from build123d import *

# Parameters (mm, degrees)
F0_W     = 15
F0_H     = 15
F0_R     = 4.955
F1_DEPTH = 7.5
F2_R     = 2.5
F3_DEPTH = 1.5
F4_R     = 2.5
F5_DEPTH = 1.5
F6_R     = 2.5
F7_DEPTH = 1.5
F8_R     = 2.5
F9_DEPTH = 1.5


with BuildPart() as f1:
    # F0 (on Top) → F1 (new body, symmetric)
    with BuildSketch(Plane.XY):
        Rectangle(F0_W, F0_H)
        Circle(F0_R, mode=Mode.SUBTRACT)
    extrude(amount=F1_DEPTH, both=True)

    # F2 (on face) → F3 (join)
    with BuildSketch(Plane(origin=(0, 7.5, 0), x_dir=(-1, 0, 0), z_dir=(0, 1, 0))):
        Circle(F2_R)
    extrude(amount=F3_DEPTH)

    # F4 (on face) → F5 (cut)
    with BuildSketch(Plane.XZ.offset(7.5)):
        Circle(F4_R)
    extrude(amount=-F5_DEPTH, mode=Mode.SUBTRACT)

    # F6 (on face) → F7 (cut)
    with BuildSketch(Plane.YZ.offset(7.5)):
        Circle(F6_R)
    extrude(amount=-F7_DEPTH, mode=Mode.SUBTRACT)

    # F8 (on face) → F9 (cut)
    with BuildSketch(Plane(origin=(-7.5, 0, 0), x_dir=(0, -1, 0), z_dir=(-1, 0, 0))):
        Circle(F8_R)
    extrude(amount=-F9_DEPTH, mode=Mode.SUBTRACT)


solid = f1.part
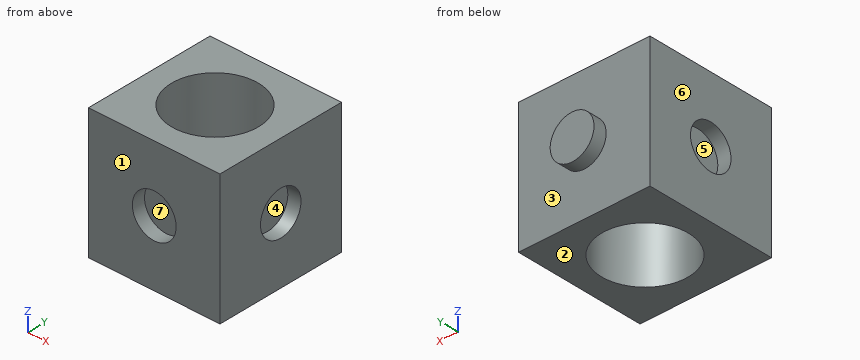
Read the model definition and answer for the solid it produces. Units are mm, in the model's axes. Face numbers are marked on the shaded views. A direction names the side the tool comes from. Coordinates: 2 decimals unless noted, no trailing zeros. Order: outer loops, then holes, each group sorted by start corner. A loop starts at its lowest first (then second) coordinate and runs counter-clockwise, first axis right, second up. Notation, with made-up numbers: M 35,-24.75 L 71,-24.75 A5 cw 71,-20.75 Z; hole C 83.25,88.25 d3. An arc over 180 degrees is marked long. Put each result on its own line as item: value. Start each with the question number.
Item 1: For the marked faces 5, 6 and 7, determine the directions among +Z, -Z, +X, -X, +Y, -Y from which every point of the face is accessible in a straight line to the end or side of a thin tool.
Item 2: Given pin 1 Ø4 at (y, z) = (0, 0) entering from +X; pin 2 Ø9 at (x, y) = (0, 0) entering from +Z; pin 3 Ø1 at (x, z) = (-3.5, -4.5) entering from +Y; pin 4 Ø1.5 at (y, z) = (1, 0.5) entering from -X, each flat-ended and moving along its own axis, determine where each tip first touches the part or whether it passes through.
Item 3: Section B-B, the plane y = 0 is taken. Determine the outline of the cut face in (x, z) (3 decimals).
Item 4: Section D-D, the plane y = -3 is taken. Determine the outline of the cut face in (x, z), plus the area to 3 significant figures.
Item 5: Section C-C, the plane x = 0 is taken. Determine the outline of the cut face in (y, z) (3 decimals), plus the area to 4 significant figures.
Item 6: Section A-A, the plane z = 0 is taken. Determine the outline of the cut face in (x, y) (3 decimals), plus the area to 3 significant figures.
Item 7: The mould has two halves that part along Y. Classify the marked faces 1, 2, 3 and 4: +Y half, -Y half, draft (parallel to the pull), parting line (faces both ways), or undercut.
Item 8: Consider probe 1 along Z at (x, y) = (-6.8, 0); probe 2 along Y at (x, z) = (0, -2) (3 decimals); probe 3 along X at (y, z) = (1.75, -0.25). Determine where each line is inside the solid, lowest interval first. Write a range as [from, to].
Computed:
1. face 5: -X
1. face 6: +Z, -Z, -X, +Y, -Y
1. face 7: -Y
2. pin 1: stops at x = 6
2. pin 2: passes through
2. pin 3: stops at y = 7.5
2. pin 4: stops at x = -6
3. outline: M -7.5,-7.5 L -4.955,-7.5 L -4.955,7.5 L -7.5,7.5 L -7.5,2.5 L -6,2.5 L -6,-2.5 L -7.5,-2.5 Z; M 4.955,-7.5 L 7.5,-7.5 L 7.5,-2.5 L 6,-2.5 L 6,2.5 L 7.5,2.5 L 7.5,7.5 L 4.955,7.5 Z
4. outline: M -7.5,-7.5 L -3.94,-7.5 L -3.94,7.5 L -7.5,7.5 Z; M 3.94,-7.5 L 7.5,-7.5 L 7.5,7.5 L 3.94,7.5 Z
4. area: 107 mm2
5. outline: M -7.5,-7.5 L -4.955,-7.5 L -4.955,7.5 L -7.5,7.5 L -7.5,2.5 L -6,2.5 L -6,-2.5 L -7.5,-2.5 Z; M 4.955,-7.5 L 7.5,-7.5 L 7.5,-2.5 L 9,-2.5 L 9,2.5 L 7.5,2.5 L 7.5,7.5 L 4.955,7.5 Z
5. area: 76.35 mm2
6. outline: M -7.5,-7.5 L -2.5,-7.5 L -2.5,-6 L 2.5,-6 L 2.5,-7.5 L 7.5,-7.5 L 7.5,-2.5 L 6,-2.5 L 6,2.5 L 7.5,2.5 L 7.5,7.5 L 2.5,7.5 L 2.5,9 L -2.5,9 L -2.5,7.5 L -7.5,7.5 L -7.5,2.5 L -6,2.5 L -6,-2.5 L -7.5,-2.5 Z; hole C 0,0 d9.91
6. area: 133 mm2
7. face 1: -Y half
7. face 2: draft
7. face 3: +Y half
7. face 4: undercut
8. probe 1: z = [-7.5, -2.5], [2.5, 7.5]
8. probe 2: y = [-6, -4.955], [4.955, 9]
8. probe 3: x = [-6, -4.64], [4.64, 6]
